The drawing under review shows one solid part. Ordinate dimensions are in mm from its lowest x, y, z. Coordinates: 2 decimals unless noted, no trailing zeros. Loops run counter-clockwise (first coordinate to the right, second up) from the corner with the lowest first, then second, coordinate; pieces in that order, holes last.
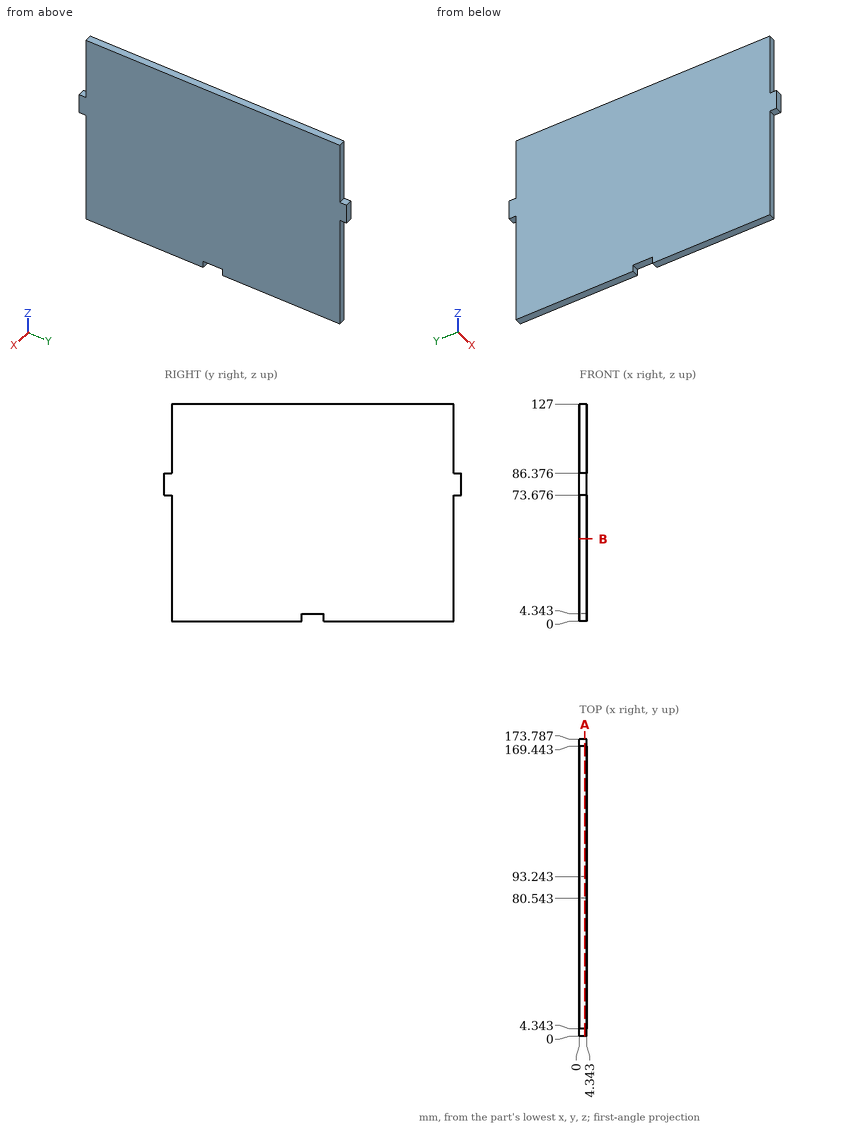
Q1. Take a section at B-B, the plane z = 48. Write out the cut boundary in (x, y).
Q2. For line 1 (Y direction, x = 0.6, z = 104); line 2 (Z direction, x = 0.85, y = 86), list the stretches that pass through material, from the lowest coordinate up.
Q3. Take a section at A-A, the plane x = 3.3. Write out the cut boundary in (y, z), then the cut area to 3 significant figures.
Q4. Clearance check with flat-ended pins moving along their axes: pin 1 Ø2 at (x, y) = (2, 3) entering from +Z; pin 2 Ø2 at (x, z) = (2, 30.5) entering from -Y; pin 3 Ø2 at (x, z) = (2.5, 24.5) entering from +Y. State where each tip first meets the part, or that it passes through.
Entries:
1. outline: (0, 4.34) - (4.34, 4.34) - (4.34, 169.44) - (0, 169.44) - close
2. line 1: y = 4.34 to 169.44
2. line 2: z = 4.34 to 127
3. outline: (0, 73.68) - (4.34, 73.68) - (4.34, 0) - (80.54, 0) - (80.54, 4.34) - (93.24, 4.34) - (93.24, 0) - (169.44, 0) - (169.44, 73.68) - (173.79, 73.68) - (173.79, 86.38) - (169.44, 86.38) - (169.44, 127) - (4.34, 127) - (4.34, 86.38) - (0, 86.38) - close
3. area: 21,000 mm2
4. pin 1: stops at z = 86.38
4. pin 2: stops at y = 4.34
4. pin 3: stops at y = 169.44
